```python
from build123d import *

# Parameters (mm, degrees)
ESQUISSE1_R             = 12.375
BOSS_EXTRU_1_DEPTH      = 50
CONG_2_R                = 5
ESQUISSE2_R             = 1.5
ENL_V_MAT_EXTRU_1_DEPTH = 51


with BuildPart() as part:
    # Esquisse1 → Boss.-Extru.1 (new body)
    with BuildSketch(Plane.XY):
        Circle(ESQUISSE1_R)
    extrude(amount=BOSS_EXTRU_1_DEPTH)

    # Congé2
    cong_2_edges = [part.edges().sort_by_distance(p)[0] for p in [
        (-12.375, 0, 50),
    ]]
    fillet(cong_2_edges, radius=CONG_2_R)

    # Esquisse2 → Enlèv. mat.-Extru.1 (cut, through all)
    with BuildSketch(Plane(origin=(0, 0, 0), x_dir=(-1, 0, 0), z_dir=(0, 0, -1))):
        Circle(ESQUISSE2_R)
    extrude(amount=-ENL_V_MAT_EXTRU_1_DEPTH, mode=Mode.SUBTRACT)


solid = part.part
```
Geometry: final body of the model. Coordinates: model frame, mm. Coordinates: 2 decimals unless noted, no trailing zeros. Write each loop counter-clockwise with the first axis right and the second up, starting at its lowest first coordinate (ties: lowest second). Pieces come first, ordered by that corner, then holes. Notation, with made-up numbers: M 77.5,24 L 93.5,24 A35 cw 93.5,62 Z; hole C -25.75,59.25 d5. An arc over 180 degrees is marked long. Use CSV: the item, a comma, the result in double quotes. Start each with the question number.
1. Mould query, pull axis Y, two halves, no side actions, for faces 1 (the face through (1.5, 0.07, 24.65)), 2 (the face through (-1.61, 12.27, 22.18)), 3 (the face through (0, -2, 50)). Classes: pulls with the +Y half, pulls with the -Y half, needs draft (parallel to the pull), parting line crosses it, or undercut.
2. First-contact query: P1, Ø8, axis at y = 7, z = 17.5, coming from the -X side; P2, Ø1, axis at x = -6.5, z = 27, coming from the +Y side; P3, Ø3, axis at y = 3.5, z = 24, coming from the +X side. Flat tips, straight axial feed; report the tip coordinate or a pass-through.
3. Cut plane C-C on z = 44.5. Return the cut outline in (x, y) (3 decimals), plus the area to 3 significant figures.
4. Ray query, probe 1 along Y at (x, z) = (0, 23.5) (3 decimals); probe 2 along Y at (x, z) = (-1.25, 34.5). Return the intervals inside material, ascending.
5. Cut plane A-A on y = 0. Return the cut outline in (x, z) (3 decimals), plus the area to 3 significant figures.
Entries:
1,face 1,"undercut"
1,face 2,"parting line crosses it"
1,face 3,"needs draft"
2,P1,"x = -12.01"
2,P2,"y = 10.82"
2,P3,"x = 12.21"
3,outline,"C 0,0 d24.75; hole C 0,0 d3"
3,area,"474 mm²"
4,probe 1,"-12.375 to -1.5, 1.5 to 12.375"
4,probe 2,"-12.31 to -0.83, 0.83 to 12.31"
5,outline,"M -12.375,0 L -1.5,0 L -1.5,50 L -7.375,50 A5 ccw -12.375,45 Z; M 1.5,0 L 12.375,0 L 12.375,45 A5 ccw 7.375,50 L 1.5,50 Z"
5,area,"1,080 mm²"
